Model file for the job. Use its own axes, mm. Face numbers are marked on the shaded views. A direction names the side the tool comes from. Give positions to 0.01 mm unless a question says otherwise; leave off trailing zeros. Loops run counter-clockwise (first coordinate to the right, second up) from the corner with the lowest first, then second, coordinate; pieces in that order, holes last. Notation, with made-up numbers: (-29, 14.5) - (10, 14.5) arc R26 cw to (10, 42.5) - close; hole circle Ø5 at (77.5, 77). An arc over 180 degrees is marked (long way). Use a Markdown table: item, result.
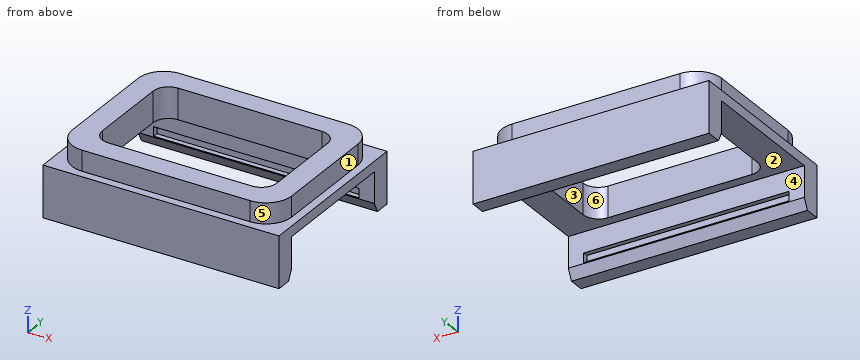
from build123d import *

# Parameters (mm, degrees)
F0_W         = 23
F0_H         = 17
F1_DEPTH     = 1
F2_DEPTH     = 3
F4_DEPTH     = 4
F5_DEPTH     = 2
F6_DEPTH     = 2
F7_W         = 1.5
F7_H         = 2
F8_DEPTH     = 4
F9_W         = 20
F9_H         = 1.1
F10_DEPTH    = 0.5
F11_W        = 20
F11_H        = 1.1
F12_DEPTH    = 0.5
F13_C1_SIZE2 = 1
F13_C1_SIZE  = 0.5
F13_C2_SIZE2 = 0.5
F13_C2_SIZE  = 1
F15_W        = 17
F15_H        = 11
F16_DEPTH    = 25
F17_R        = 1.5


# Not quite as in the source:
# - two fillets or chamfers of one size are made in one step


with BuildPart() as f1:
    # F0 (on Top) → F1 (new body)
    with BuildSketch(Plane.XY):
        Rectangle(F0_W, F0_H)
        with BuildLine():
            Line((-8.2, 7.7), (8.2, 7.7))
            ThreePointArc((8.2, 7.7), (9.967766953, 6.967766953), (10.7, 5.2))
            Line((10.7, 5.2), (10.7, -5.2))
            ThreePointArc((10.7, -5.2), (9.967766953, -6.967766953), (8.2, -7.7))
            Line((8.2, -7.7), (-8.2, -7.7))
            ThreePointArc((-8.2, -7.7), (-9.967766953, -6.967766953), (-10.7, -5.2))
            Line((-10.7, -5.2), (-10.7, 5.2))
            ThreePointArc((-10.7, 5.2), (-9.967766953, 6.967766953), (-8.2, 7.7))
        make_face(mode=Mode.SUBTRACT)
    extrude(amount=F1_DEPTH)

    # F0 (on Top) → F2 (join)
    with BuildSketch(Plane.XY):
        with BuildLine():
            ThreePointArc((10.7, 5.2), (9.967766953, 6.967766953), (8.2, 7.7))
            Line((8.2, 7.7), (-8.2, 7.7))
            ThreePointArc((-8.2, 7.7), (-9.967766953, 6.967766953), (-10.7, 5.2))
            Line((-10.7, 5.2), (-10.7, -5.2))
            ThreePointArc((-10.7, -5.2), (-9.967766953, -6.967766953), (-8.2, -7.7))
            Line((-8.2, -7.7), (8.2, -7.7))
            ThreePointArc((8.2, -7.7), (9.967766953, -6.967766953), (10.7, -5.2))
            Line((10.7, -5.2), (10.7, 5.2))
        make_face()
    extrude(amount=F2_DEPTH)

    # F3 (on face) → F4 (join)
    with BuildSketch(Plane.XY):
        with BuildLine():
            Line((10, -8.5), (10, -7))
            Line((10, -7), (9.9349351573, -7))
            ThreePointArc((9.9349351573, -7), (9.1354143467, -7.5184046239), (8.2, -7.7))
            Line((8.2, -7.7), (-8.2, -7.7))
            ThreePointArc((-8.2, -7.7), (-9.1354143467, -7.5184046239), (-9.9349351573, -7))
            Line((-9.9349351573, -7), (-10, -7))
            Line((-10, -7), (-10, -8.5))
            Line((-10, -8.5), (10, -8.5))
        make_face()
        with BuildLine():
            ThreePointArc((8.2, -7.7), (9.1354143467, -7.5184046239), (9.9349351573, -7))
            Line((9.9349351573, -7), (-9.9349351573, -7))
            ThreePointArc((-9.9349351573, -7), (-9.1354143467, -7.5184046239), (-8.2, -7.7))
            Line((-8.2, -7.7), (8.2, -7.7))
        make_face()
        with BuildLine():
            Line((9.9349351573, 7), (10, 7))
            Line((10, 7), (10, 8.5))
            Line((10, 8.5), (-10, 8.5))
            Line((-10, 8.5), (-10, 7))
            Line((-10, 7), (-9.9349351573, 7))
            ThreePointArc((-9.9349351573, 7), (-9.1354143467, 7.5184046239), (-8.2, 7.7))
            Line((-8.2, 7.7), (8.2, 7.7))
            ThreePointArc((8.2, 7.7), (9.1354143467, 7.5184046239), (9.9349351573, 7))
        make_face()
        with BuildLine():
            Line((-9.9349351573, 7), (9.9349351573, 7))
            ThreePointArc((9.9349351573, 7), (9.1354143467, 7.5184046239), (8.2, 7.7))
            Line((8.2, 7.7), (-8.2, 7.7))
            ThreePointArc((-8.2, 7.7), (-9.1354143467, 7.5184046239), (-9.9349351573, 7))
        make_face()
    extrude(amount=-F4_DEPTH)

    # F3 (on face) → F5 (join)
    with BuildSketch(Plane.XY):
        with BuildLine():
            Line((-9.9349351573, -7), (9.9349351573, -7))
            ThreePointArc((9.9349351573, -7), (9.967766953, -6.967766953), (10, -6.9349351573))
            Line((10, -6.9349351573), (10, -6.5))
            Line((10, -6.5), (-10, -6.5))
            Line((-10, -6.5), (-10, -6.9349351573))
            ThreePointArc((-10, -6.9349351573), (-9.967766953, -6.967766953), (-9.9349351573, -7))
        make_face()
        with BuildLine():
            Line((10, 6.5), (10, 6.9349351573))
            ThreePointArc((10, 6.9349351573), (9.967766953, 6.967766953), (9.9349351573, 7))
            Line((9.9349351573, 7), (-9.9349351573, 7))
            ThreePointArc((-9.9349351573, 7), (-9.967766953, 6.967766953), (-10, 6.9349351573))
            Line((-10, 6.9349351573), (-10, 6.5))
            Line((-10, 6.5), (10, 6.5))
        make_face()
    extrude(amount=-F5_DEPTH)

    # F3 (on face) → F6 (join)
    with BuildSketch(Plane.XY):
        with BuildLine():
            Line((9.9349351573, -7), (10, -7))
            Line((10, -7), (10, -6.9349351573))
            ThreePointArc((10, -6.9349351573), (9.967766953, -6.967766953), (9.9349351573, -7))
        make_face()
        with BuildLine():
            Line((-10, -7), (-9.9349351573, -7))
            ThreePointArc((-9.9349351573, -7), (-9.967766953, -6.967766953), (-10, -6.9349351573))
            Line((-10, -6.9349351573), (-10, -7))
        make_face()
        with BuildLine():
            ThreePointArc((9.9349351573, 7), (9.967766953, 6.967766953), (10, 6.9349351573))
            Line((10, 6.9349351573), (10, 7))
            Line((10, 7), (9.9349351573, 7))
        make_face()
        with BuildLine():
            Line((-10, 7), (-10, 6.9349351573))
            ThreePointArc((-10, 6.9349351573), (-9.967766953, 6.967766953), (-9.9349351573, 7))
            Line((-9.9349351573, 7), (-10, 7))
        make_face()
    extrude(amount=-F6_DEPTH)

    # F7 (on face) → F8 (join)
    with BuildSketch(Plane(origin=(0, 0, 0), x_dir=(1, 0, 0), z_dir=(0, 0, -1))):
        with Locations((10.75, 7.5)):
            Rectangle(F7_W, F7_H)
        with Locations((-10.75, 7.5)):
            Rectangle(F7_W, F7_H)
        with Locations((-10.75, -7.5)):
            Rectangle(F7_W, F7_H)
        with Locations((10.75, -7.5)):
            Rectangle(F7_W, F7_H)
    extrude(amount=F8_DEPTH)

    # F9 (on face) → F10 (join)
    with BuildSketch(Plane(origin=(0, -7, 0), x_dir=(-1, 0, 0), z_dir=(0, 1, 0))):
        with Locations((0, -3.45)):
            Rectangle(F9_W, F9_H)
    extrude(amount=F10_DEPTH)

    # F11 (on face) → F12 (join)
    with BuildSketch(Plane.XZ.offset(-7)):
        with Locations((0, -3.45)):
            Rectangle(F11_W, F11_H)
    extrude(amount=F12_DEPTH)

    # F13: chamfer of 0.5 x 1 on 2 edges, made by hand

    # F13_c1
    f13_c1_edges = [f1.edges().sort_by_distance(p)[0] for p in [
        (0, -6.5, -4),
    ]]
    f13_c1_side = f1.faces().sort_by_distance((0, -6.51, -4))[0]
    chamfer(f13_c1_edges, length=F13_C1_SIZE, length2=F13_C1_SIZE2, reference=f13_c1_side)

    # F13_c2
    f13_c2_edges = [f1.edges().sort_by_distance(p)[0] for p in [
        (0, 6.5, -4),
    ]]
    f13_c2_side = f1.faces().sort_by_distance((0, 6.5, -3.99))[0]
    chamfer(f13_c2_edges, length=F13_C2_SIZE, length2=F13_C2_SIZE2, reference=f13_c2_side)

    # F15 (on face) → F16 (cut)
    with BuildSketch(Plane.XY.offset(3)):
        Rectangle(F15_W, F15_H)
    extrude(amount=-F16_DEPTH, mode=Mode.SUBTRACT)

    # F17
    f17_edges = [f1.edges().sort_by_distance(p)[0] for p in [
        (-8.5, -5.5, 1.5),
        (-8.5, 5.5, 1.5),
        (8.5, 5.5, 1.5),
        (8.5, -5.5, 1.5),
    ]]
    fillet(f17_edges, radius=F17_R)


solid = f1.part
(1) Drill centre lines: probe 1 along Y at (x, z) = (-6.25, 0.25); probe 2 along X at (y, z) = (-1.25, 1.75); probe 3 along Y at (x, z) = (1.25, -1). Where is each one in solid material? Low to high. Write a range as [from, to].
Computed:
| item | result |
|---|---|
| probe 1 | [-8.5, -5.5], [5.5, 8.5] |
| probe 2 | [-10.7, -8.5], [8.5, 10.7] |
| probe 3 | [-8.5, -6.5], [6.5, 8.5] |
(2) Slice it at A-A, the plane y = 3.75. Write the cut outline in (x, z).
Computed:
| item | result |
|---|---|
| outline | (-11.5, 0) - (-8.5, 0) - (-8.5, 3) - (-10.7, 3) - (-10.7, 1) - (-11.5, 1) - close; (8.5, 0) - (11.5, 0) - (11.5, 1) - (10.7, 1) - (10.7, 3) - (8.5, 3) - close |
(3) Pin check, flat tips, straight feed: P1, Ø1, axis at y = 3, z = -2, coming from the -X side; P2, Ø0.6, axis at x = -1, y = 6.5, coming from the -Z side; P3, Ø0.6, axis at y = 0, z = 2, coming from the -X side; P4, Ø0.6, axis at x = 3, z = 2, coming from the +Y side. Stop position of each tip, or through.
Computed:
| item | result |
|---|---|
| P1 | through |
| P2 | z = -3.6 |
| P3 | x = -10.7 |
| P4 | y = 7.7 |
(4) Slice it at D-D, the plane z = 2. Write the cut outline in (x, y), plus the area to 3 significant figures.
Computed:
| item | result |
|---|---|
| outline | (-10.7, -5.2) arc R2.5 ccw to (-8.2, -7.7) - (8.2, -7.7) arc R2.5 ccw to (10.7, -5.2) - (10.7, 5.2) arc R2.5 ccw to (8.2, 7.7) - (-8.2, 7.7) arc R2.5 ccw to (-10.7, 5.2) - close; hole (-8.5, -4) arc R1.5 ccw to (-7, -5.5) - (7, -5.5) arc R1.5 ccw to (8.5, -4) - (8.5, 4) arc R1.5 ccw to (7, 5.5) - (-7, 5.5) arc R1.5 ccw to (-8.5, 4) - close |
| area | 139 mm² |
(5) Slice it at B-B, the plane z = -2.5. Write the cut outline in (x, y).
Computed:
| item | result |
|---|---|
| outline | (-11.5, -8.5) - (11.5, -8.5) - (11.5, -6.5) - (10, -6.5) - (10, -7) - (-10, -7) - (-10, -6.5) - (-11.5, -6.5) - close; (-11.5, 6.5) - (-10, 6.5) - (-10, 7) - (10, 7) - (10, 6.5) - (11.5, 6.5) - (11.5, 8.5) - (-11.5, 8.5) - close |
(6) Mould opens along X. For the marked faces 1, 2 and 3 say: pulls with the +X half, pulls with the -X half, needs draft (parallel to the pull), parting line crosses it, or undercut.
Computed:
| item | result |
|---|---|
| face 1 | pulls with the +X half |
| face 2 | needs draft |
| face 3 | undercut |
(7) 3-axis set-ups, long thin cutter, end or side, ignore diameter. For the marked faces 4, 5 and 6: which of +Z, -Z, +X, -X, +Y, -Y reach the whole face in a straight line?
Computed:
| item | result |
|---|---|
| face 4 | -Z, +X, -X |
| face 5 | +Z, +X, -Y |
| face 6 | +Z, -Z |
(8) Slice it at C-C, the plane x = 0.5. Write the cut outline in (y, z).
Computed:
| item | result |
|---|---|
| outline | (-8.5, -4) - (-7, -4) - (-6.5, -3) - (-6.5, -2.9) - (-7, -2.9) - (-7, -2) - (-6.5, -2) - (-6.5, 0) - (-5.5, 0) - (-5.5, 3) - (-7.7, 3) - (-7.7, 1) - (-8.5, 1) - close; (5.5, 0) - (6.5, 0) - (6.5, -2) - (7, -2) - (7, -2.9) - (6.5, -2.9) - (6.5, -3) - (7, -4) - (8.5, -4) - (8.5, 1) - (7.7, 1) - (7.7, 3) - (5.5, 3) - close |
